```python
from build123d import *

# Parameters (mm, degrees)
BOSS_EXTRUDE1_DEPTH = 1.5875
CUT_EXTRUDE1_DEPTH  = 3.175
FILLET1_R           = 8.89


with BuildPart() as part:
    # Sketch1 → Boss-Extrude1 (new, symmetric)
    with BuildSketch(Plane.XY):
        with BuildLine():
            Line((-127.293308919, -32.555250036), (-85.984130762, -73.864428193))
            Line((-85.984130762, -73.864428193), (-85.984130762, -86.643760402))
            ThreePointArc((-85.984130762, -86.643760402), (-70.818680903, -97.099597285), (-54.399250036, -105.449308919))
            ThreePointArc((-54.399250036, -105.449308919), (97.88479172, 119.72879172), (-127.293308919, -32.555250036))
        make_face()
    extrude(amount=BOSS_EXTRUDE1_DEPTH, both=True)

    # Sketch2 → Cut-Extrude1 (cut)
    with BuildSketch(Plane.XY.offset(1.5875)):
        with BuildLine():
            Line((-114.372852664, -23.923091601), (-70.744130762, -67.551813503))
            Line((-70.744130762, -67.551813503), (-70.744130762, -79.00759425))
            ThreePointArc((-70.744130762, -79.00759425), (96.569405073, 98.330117066), (-114.372852664, -23.923091601))
        make_face()
    extrude(amount=-CUT_EXTRUDE1_DEPTH, mode=Mode.SUBTRACT)

    # Fillet1
    fillet1_edges = [part.edges().sort_by_distance(p)[0] for p in [
        (-114.372852664, -23.923091601, 0),
        (-70.744130762, -79.00759425, 0),
        (-70.744130762, -67.551813503, 0),
        (-85.984130762, -86.643760402, -0.79375),
        (-85.984130762, -73.864428193, -0.79375),
        (-127.293308919, -32.555250036, -0.79375),
    ]]
    fillet(fillet1_edges, radius=FILLET1_R)


solid = part.part
```
Source: CAD feature listing. Evaluate the final solid. Frame: model axes, mm. A direction names the side the tool comes from. Round coordinates to 2 decimals unless told otherwise and drop trailing zeros. Loops run counter-clockwise (first coordinate to the right, second up) from the corner with the lowest first, then second, coordinate; pieces in that order, holes last. Notation, with made-up numbers: M 2.25,42 L 53.25,42 A31 ccw 53.25,73 Z; hole C 39,-24.75 d5. An arc over 180 degrees is marked long. Use a Markdown table: item, result. Add a question column.
1. Pull-direction query (X, two-part tool) for faces 1 (the cylindrical face through (98.631, 95.653, 0.022)), 2 (the flat face through (-107.59, -52.26, 0.02)), 3 (the flat face through (-83, -60, 1.588)); classes: +X half, -X half, draft (parallel to the pull), parting line (faces both ways), or undercut.
2. Contact query for a flat-ended pin moving along its axis: pin 1 (1 mm diameter, centred on y = -80, z = 0, fed in from -X). Output: stop coordinate, or through.
3. Set-up query: faces 4 (the flat face through (-93.481, -44.815, 0.022)), 5 (the flat face through (-83, -60, -1.588)). Return all of +Z, -Z, +X, -X, +Y, -Y with unobstructed straight access to the full face (end or side cutting, diameter ignored); none if empty.
4. Cut plane B-B, the plane z = -0.1. Output: boundary loops of the cut face in (x, y) (3 decimals), and give its area (3 significant figures).
5. Cut plane A-A, the plane x = 0. Output: boundary loops of the cut face in (y, z).
6. Ray query, line 1 along Y through (x, z) = (1.5, -1.3); line 2 along Y through (x, z) = (-49.5, 0.8); line 3 along X through (y, z) = (93, 1). Return the intervals inside material, ascending. Write a range as [from, to].
7. Cut plane C-C, the plane y = 42. Output: boundary loops of the cut face in (x, z), and give its area (3 significant figures).
Solution:
| question | item | result |
|---|---|---|
| 1 | face 1 | undercut |
| 1 | face 2 | -X half |
| 1 | face 3 | draft |
| 2 | pin 1 | stops at x = -85.98 |
| 3 | face 4 | +Z, -Z |
| 3 | face 5 | -Z, +X, -X, +Y, -Y |
| 4 | outline | M -127.992,-30.891 A8.89 ccw -126.058,-33.79 L -88.588,-71.261 A8.89 cw -85.984,-77.547 L -85.984,-82.257 A8.89 ccw -82.385,-89.402 A138.43 ccw long Z; hole M -115.076,-22.125 A8.89 ccw -113.058,-25.238 L -73.348,-64.948 A8.89 cw -70.744,-71.234 L -70.744,-74.273 A8.89 ccw -66.665,-81.749 A123.19 ccw long Z |
| 4 | area | 12,600 mm2 |
| 5 | outline | M -116.59,-1.59 L -101.35,-1.59 L -101.35,1.59 L -116.59,1.59 Z; M 145.03,-1.59 L 160.27,-1.59 L 160.27,1.59 L 145.03,1.59 Z |
| 6 | line 1 | y = [-116.58, -101.34], [145.02, 160.27] |
| 6 | line 2 | y = [-107.43, -90.96], [134.65, 151.12] |
| 6 | line 3 | x = [-118.74, -100.56], [100.56, 118.74] |
| 7 | outline | M -136.95,-1.59 L -121.53,-1.59 L -121.53,1.59 L -136.95,1.59 Z; M 121.53,-1.59 L 136.95,-1.59 L 136.95,1.59 L 121.53,1.59 Z |
| 7 | area | 97.9 mm2 |
